Geometry check sheet. Reference: the model listing, model coordinates, mm. A direction names the side the tool comes from. Round coordinates to 2 decimals unless told otherwise and drop trailing zeros. Order: outer loops, then holes, each group sorted by start corner. A loop starts at its lowest first (then second) coordinate and runs counter-clockwise, first axis right, second up.
(1) Sectioned sample at A-A (z = 9). Record the boundary of the cut face in (x, y), plus the area to 3 significant figures.
(2) Sectioned sample at B-B (x = -5). Record the boundary of the cut face in (y, z) (3 decimals), plus the area to 3 significant figures.
(3) Material ranges on line 1 along X through (y, z) = (12, 1.5) (3 decimals); line 2 along Z through (x, y) = (-5.39, 0.7); line 3 along Y through (x, z) = (-6.25, 2.5), recorded low to high.
(4) Sectioned sample at C-C (y = 5.25). Record the boundary of the cut face in (x, z), plus the area to 3 significant figures.
(5) Go/stop test with a flat-tipped pin: pin 1 (6 mm diameter, centred on x = -3, y = 9.5, fed in from +Z). Record where the tip stops, or that it passes through.
(6) Set-up check for faces 1 (the face through (-12, 2, 7)), 2 (the face through (-25, 8.7, 1.6)), 3 (the face through (-4.931, 22.124, 1.014)): record each of +Z, -Z, +X, -X, +Y, -Y from which the full face is reachable in a straight line by a thin tool's end or side.
(7) Release check for a two-part mould opening along Z. For faces 4 (the face through (-12, 0, 6)), 5 (the face through (-12, 14, 2)), 6 (the face through (-20.996, 1.014, 8.425)) record: +Z half, -Z half, draft (parallel to the pull), parting line (faces both ways), or undercut.
(8) Sectioned sample at D-D (x = -23.5). Record the boundary of the cut face in (y, z), plus the area to 3 significant figures.
from build123d import *

# Parameters (mm, degrees)
F1_DEPTH = 25
F2_R     = 1.5
F3_DEPTH = 25
F5_DEPTH = 25


with BuildPart() as f1:
    # F0 (on Right) → F1 (new body)
    with BuildSketch(Plane.YZ):
        Polygon((0, 12), (0, 0), (25, 0), (25, 2), (2, 2), (2, 12), align=None)
    extrude(amount=-F1_DEPTH)

    # F2 (on face) → F3 (cut)
    with BuildSketch(Plane(origin=(0, 2, 0), x_dir=(-1, 0, 0), z_dir=(0, 1, 0))):
        with Locations((5.39, 9)):
            Circle(F2_R)
        with Locations((19.61, 9)):
            Circle(F2_R)
    extrude(amount=-F3_DEPTH, mode=Mode.SUBTRACT)

    # F4 (on face) → F5 (cut)
    with BuildSketch(Plane.XY.offset(2)):
        with BuildLine():
            Line((-16.875, 11), (-16.875, 19))
            ThreePointArc((-16.875, 19), (-20, 22.125), (-23.125, 19))
            Line((-23.125, 19), (-23.125, 11))
            ThreePointArc((-23.125, 11), (-20, 7.875), (-16.875, 11))
        make_face()
        with BuildLine():
            Line((-1.875, 11), (-1.875, 19))
            ThreePointArc((-1.875, 19), (-5, 22.125), (-8.125, 19))
            Line((-8.125, 19), (-8.125, 11))
            ThreePointArc((-8.125, 11), (-5, 7.875), (-1.875, 11))
        make_face()
    extrude(amount=-F5_DEPTH, mode=Mode.SUBTRACT)


solid = f1.part
Answer below:
1. outline: (-25, 0) - (-21.11, 0) - (-21.11, 2) - (-25, 2) - close; (-18.11, 0) - (-6.89, 0) - (-6.89, 2) - (-18.11, 2) - close; (-3.89, 0) - (0, 0) - (0, 2) - (-3.89, 2) - close
1. area: 38.0 mm2
2. outline: (0, 0) - (7.875, 0) - (7.875, 2) - (2, 2) - (2, 7.552) - (0, 7.552) - close; (0, 10.448) - (2, 10.448) - (2, 12) - (0, 12) - close; (22.125, 0) - (25, 0) - (25, 2) - (22.125, 2) - close
2. area: 35.7 mm2
3. line 1: x = -25 to -23.125, -16.875 to -8.125, -1.875 to 0
3. line 2: z = 0 to 7.5, 10.5 to 12
3. line 3: y = 0 to 2
4. outline: (-25, 0) - (0, 0) - (0, 2) - (-25, 2) - close
4. area: 50.0 mm2
5. pin 1: stops at z = 2
6. face 1: +Z, +X, -X, +Y
6. face 2: +Z, -Z, -X, +Y, -Y
6. face 3: +Z, -Z
7. face 4: draft
7. face 5: +Z half
7. face 6: undercut
8. outline: (0, 0) - (25, 0) - (25, 2) - (2, 2) - (2, 12) - (0, 12) - close
8. area: 70.0 mm2
